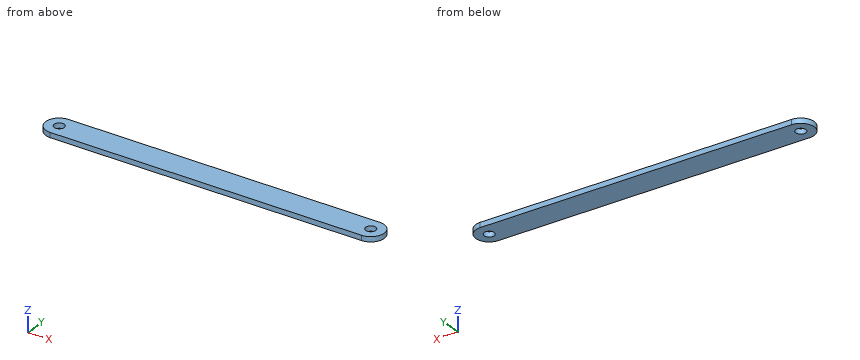
```python
from build123d import *

# Parameters (mm, degrees)
SKETCH_1_R      = 8
SKETCH_1_R_2    = 3
EXTRUDE_1_DEPTH = 3


with BuildPart() as part:
    # 草图1 → 凸台-拉伸1 (new body)
    # profile 1 of 3: a face of its own
    with BuildSketch(Plane.XY):
        with BuildLine():
            Line((92.999999991, 8), (-93, 8))
            ThreePointArc((-93, 8), (-87.343145751, 5.656854249), (-85, 0))
            ThreePointArc((-85, 0), (-87.343145751, -5.656854249), (-93, -8))
            Line((-93, -8), (93.000000101, -8))
            ThreePointArc((93.000000101, -8), (85, -5.5e-08), (92.999999991, 8))
        make_face()
    # profile 2 of 3: a face of its own
    with BuildSketch(Plane.XY):
        with Locations((-93, 0)):
            Circle(SKETCH_1_R)
        with Locations((-93, 0)):
            Circle(SKETCH_1_R_2, mode=Mode.SUBTRACT)
    # profile 3 of 3: a face of its own
    with BuildSketch(Plane.XY):
        with Locations((93, 0)):
            Circle(SKETCH_1_R)
        with Locations((93, 0)):
            Circle(SKETCH_1_R_2, mode=Mode.SUBTRACT)
    extrude(amount=EXTRUDE_1_DEPTH)


solid = part.part
```
Input: part model. Units: mm. Frame: model coordinates. Give positions to 0.01 mm unless a question says otherwise; leave off trailing zeros. Order: outer loops, then holes, each group sorted by start corner. A loop starts at its lowest first (then second) coordinate and runs counter-clockwise, first axis right, second up.
1. Material intervals for L1, parallel to X at y = 2.25, z = 1.1; L2, parallel to X at y = -2, z = 2.25; L3, parallel to Y at x = -93, z = 2.3, sorted ascending.
Derived:
L1: x = -100.68 to -94.98, -91.02 to 91.02, 94.98 to 100.68
L2: x = -100.75 to -95.24, -90.76 to 90.76, 95.24 to 100.75
L3: y = -8 to -3, 3 to 8
2. Section B-B on z = 1.2. Return the cut outline in (x, y).
Derived:
outline: (-93, -8) - (93, -8) arc R8 ccw to (93, 8) - (-93, 8) arc R8 ccw to start; hole circle Ø6 at (-93, 0); hole circle Ø6 at (93, 0)
3. Pin query (flat end, axial travel): pin 1 (3.5 mm diameter, centred on x = -93, y = 0, fed in from -Z); pin 2 (3 mm diameter, centred on x = -64, y = 3, fed in from -Z). Return the tip coordinate at first contact, or that it passes through.
Derived:
pin 1: passes through
pin 2: stops at z = 0
4. Section A-A on y = 0. Return the cut outline in (x, z).
Derived:
outline: (-101, 0) - (-96, 0) - (-96, 3) - (-101, 3) - close; (-90, 0) - (90, 0) - (90, 3) - (-90, 3) - close; (96, 0) - (101, 0) - (101, 3) - (96, 3) - close
